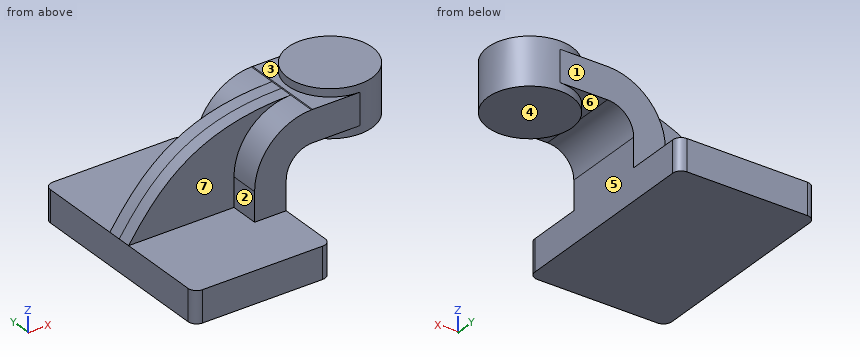
```python
from build123d import *

# Parameters (mm, degrees)
F1_DEPTH = 63.5
F2_DEPTH = 25.4
F3_DEPTH = 7.9375
F4_DEPTH = 25.4
F6_R     = 5.08
F7_R     = 5.08


with BuildPart() as f1:
    # F0 (on Front) → F1 (new body, symmetric)
    with BuildSketch(Plane.XZ):
        Polygon((22.225, 9.525), (-41.275, 9.525), (-41.275, -9.525), (41.275, -9.525), (41.275, 9.525), align=None)
    extrude(amount=F1_DEPTH, both=True)

    # F0 (on Front) → F2 (join, symmetric)
    with BuildSketch(Plane.XZ):
        with BuildLine():
            Line((22.225, 27.0002), (22.225, 9.525))
            Line((22.225, 9.525), (41.275, 9.525))
            Line((41.275, 9.525), (41.275, 27.0002))
            ThreePointArc((41.275, 27.0002), (45.92468, 38.22552), (57.15, 42.8752))
            Line((57.15, 42.8752), (60.325, 42.8752))
            Line((60.325, 42.8752), (60.325, 61.9252))
            Line((60.325, 61.9252), (57.15, 61.9252))
            add(Edge.make_bspline(
                [(56.406163, 61.917278), (56.653442, 61.920357), (56.901387, 61.922998), (57.15, 61.9252)],
                knots=[111.019471, 111.019471, 111.019471, 111.019471, 111.504536, 111.504536, 111.504536, 111.504536], degree=3))
            ThreePointArc((56.406163, 61.917278), (32.192695, 51.431503), (22.225, 27.0002))
        make_face()
    extrude(amount=F2_DEPTH, both=True)

    # F0 (on Front) → F3 (join, symmetric)
    with BuildSketch(Plane.XZ):
        with BuildLine():
            add(Edge.make_bspline(
                [(-41.275, 9.525), (-21.931022, 37.55873), (-0.190027, 61.212503), (56.406163, 61.917278)],
                knots=[0, 0, 0, 0, 111.019471, 111.019471, 111.019471, 111.019471], degree=3))
            Line((-41.275, 9.525), (22.225, 9.525))
            Line((22.225, 9.525), (22.225, 27.0002))
            ThreePointArc((22.225, 27.0002), (32.192695, 51.431503), (56.406163, 61.917278))
        make_face()
    extrude(amount=F3_DEPTH, both=True)

    # F0 (on Front) → F4 (join, symmetric)
    with BuildSketch(Plane.XZ):
        Polygon((81.447226, 61.9252), (60.325, 61.9252), (60.325, 42.8752), (81.447226, 42.8752), (85.725, 42.8752), (85.725, 61.9252), align=None)
    extrude(amount=F4_DEPTH, both=True)

    # F0 (on Front) → F5 (revolve)
    with BuildSketch(Plane.XZ):
        Polygon((111.125, 66.675), (85.725, 66.675), (85.725, 61.9252), (85.725, 42.8752), (85.725, 38.1), (111.125, 38.1), align=None)
    revolve(axis=Axis((85.725, 0, 52.3875), (0, 0, 1)))

    # F6
    f6_edges = [f1.edges().sort_by_distance(p)[0] for p in [
        (-41.275, -63.5, 0),
        (41.275, -63.5, 0),
        (41.275, 63.5, 0),
    ]]
    fillet(f6_edges, radius=F6_R)

    # F7
    f7_edges = [f1.edges().sort_by_distance(p)[0] for p in [
        (-41.275, 63.5, 0),
    ]]
    fillet(f7_edges, radius=F7_R)


solid = f1.part
```
Input: part model. Units: mm. Frame: model coordinates. Face numbers are marked on the shaded views. A direction names the side the tool comes from. Coordinates: 2 decimals unless noted, no trailing zeros. Loops run counter-clockwise (first coordinate to the right, second up) from the corner with the lowest first, then second, coordinate; pieces in that order, holes last. Notation, with made-up numbers: M -8.5,-11.75 L 14.5,-11.75 A23 cw 14.5,-2.75 Z; hole C 20.5,77 d2. An arc over 180 degrees is marked long. Use a Markdown table: item, result. Add a question column.
1) Line query: L1, parallel to X at y = 46.5, z = -1 (3 decimals); L2, parallel to Z at x = 6, y = -12.5 (3 decimals); L3, parallel to Y at x = 31, z = 31. Output: solid intervals per line, ascending. Write a range as from..to.
2) Pin query (flat end, axial travel): P1, Ø6, axis at x = 37, z = 20.5, coming from the -Y side; P2, Ø14.5, axis at x = 69.5, y = 2, coming from the -Z side; P3, Ø1.5, axis at y = -16.5, z = 6, coming from the +X side (3 decimals). Return the tip coordinate at first contact, or that it passes through.
3) Section A-A, the plane y = -28.5. Return the cut outline in (x, z) (3 decimals), plus the area to 3 significant figures.
4) Set-up query: the marked faces 1, 2, 3 and 4. Return all of +Z, -Z, +X, -X, +Y, -Y with unobstructed straight access to the full face (end or side cutting, diameter ignored); none if empty.
5) Section B-B, the plane x = 74. Return the cut outline in (y, z) (3 decimals), plus the area to 3 significant figures.
6) Draft query along X for the marked faces 5, 6 and 7. Return one class per face: +X half, -X half, draft (parallel to the pull), parting line (faces both ways), or undercut.
Answer below:
| question | item | result |
|---|---|---|
| 1 | L1 | -41.275..41.275 |
| 1 | L2 | -9.525..9.525 |
| 1 | L3 | -25.4..25.4 |
| 2 | P1 | y = -25.4 |
| 2 | P2 | z = 38.1 |
| 2 | P3 | x = 41.275 |
| 3 | outline | M -41.275,-9.525 L 41.275,-9.525 L 41.275,9.525 L -41.275,9.525 Z |
| 3 | area | 1,570 mm2 |
| 4 | face 1 | +Z, +X, -X, +Y |
| 4 | face 2 | +Z, -X, -Y |
| 4 | face 3 | +Z, -X |
| 4 | face 4 | -Z, +X, +Y, -Y |
| 5 | outline | M -25.4,42.875 L -22.532,42.875 L -22.532,38.1 L 22.532,38.1 L 22.532,42.875 L 25.4,42.875 L 25.4,61.925 L 22.532,61.925 L 22.532,66.675 L -22.532,66.675 L -22.532,61.925 L -25.4,61.925 Z |
| 5 | area | 1,400 mm2 |
| 6 | face 5 | +X half |
| 6 | face 6 | undercut |
| 6 | face 7 | draft |
